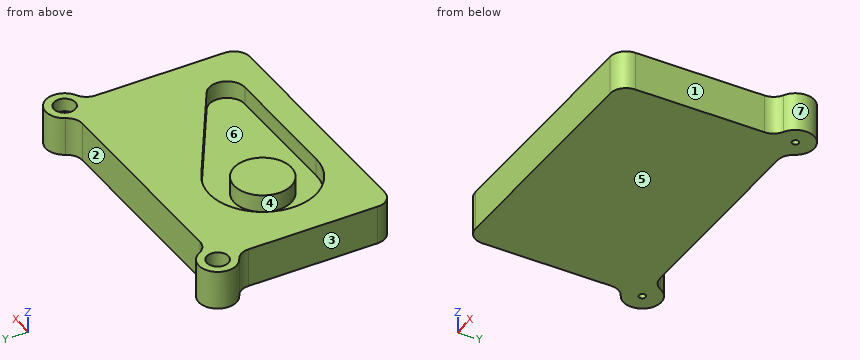
Autodesk Inventor part; units mm, degrees
ref_plane "YZ Plane" through (0, 0, 0) normal (1, 0, 0) x (0, 1, 0)
ref_plane "XZ Plane" through (0, 0, 0) normal (0, 1, 0) x (-1, 0, 0)
ref_plane "XY Plane" through (0, 0, 0) normal (0, 0, 1) x (1, 0, 0)
sketch "Sketch1" plane through (0, 0, 0) normal (0, 0, 1) x (1, 0, 0)
  line L0 (-85.9222, 66) -> (85.9222, 66)
  line L1 (100, 51.9222) -> (100, -66)
  line L2 (100, -66) -> (-100, -66)
  line L3 (-100, -66) -> (-100, 51.9222)
  line L4 (-100, 66) -> (100, -66) construction
  line L5 (100, 66) -> (-100, -66) construction
  arc A0 (-85.9222, 66) -> (-100, 51.9222) centre (-100, 66) ccw
  arc A1 (100, 51.9222) -> (85.9222, 66) centre (100, 66) ccw
  line L6 (0, 116.2908) -> (0, -96.3818)
  line L7 (-167.8726, 0) -> (167.8726, 0)
  point P0 (0, 0)
  dimension "d0" = 200
  dimension "d1" = 132
  dimension "d3" = 28.1556
  dimension "d35" = 200
extrude "Extrusion1" add sketch "Sketch1" along normal blind 29.2
fillet "Fillet1" radius 12 6 edges at (-85.9222, 66, 14.6) (85.9222, 66, 14.6) (-100, 51.9222, 14.6) (-100, -66, 14.6) (100, -66, 14.6) (100, 51.9222, 14.6)
sketch "Sketch2" plane through (0, 0, 29.2) normal (0, 0, 1) x (1, 0, 0)
  arc A0 (-87.5012, 72.4781) -> (-106.4781, 53.5012) centre (-100, 66) ccw
  circle A1 centre (-33.4, -6) radius 21.33
  arc A2 (-12.2198, 27.9323) -> (-33.4, -46) centre (-33.4, -6) ccw
  arc A3 (59.8, -46) -> (66.8424, -21.4175) centre (59.8, -32.7) ccw
  line L0 (-33.4, -46) -> (59.8, -46)
  line L1 (66.8424, -21.4175) -> (-12.2198, 27.9323)
  point P0 (-88, -66)
  point P1 (0, 0)
  dimension "d7" = 42.66
  dimension "d8" = 60
  dimension "d9" = 66.6
  dimension "d10" = 80
  dimension "d12" = 93.2
  dimension "d13" = 26.6
extrude "Extrusion2" cut sketch "Sketch2" against normal blind 13.2
hole "Hole1" at (-100, 66, 29.2) direction (0, 0, -1) diameter 5 end through all counterbore diameter 16 counterbore depth 13.2
hole "Hole2" at (100, 66, 29.2) direction (0, 0, -1) diameter 5 end through all counterbore diameter 16 counterbore depth 10
equation "\"d1\" = 0.66 * d0"
equation "\"d3\" = 0.2133 * d1"
equation "\"d35\" = d0"
equation "\"d4\" = 0.146 * d0"
equation "\"d6\" = 0.06 * d0"
equation "\"d7\" = 0.2133 * d0"
equation "\"d9\" = 0.333 * d0"
equation "\"d10\" = 0.4 * d0"
equation "\"d12\" = 0.466 * d0"
equation "\"d13\" = 0.133 * d0"
equation "\"d15\" = 0.066 * d0"
equation "\"d21\" = 0.08 * d0"
equation "\"d22\" = 0.066 * d0"
equation "\"d30\" = 0.08 * d0"
equation "\"d31\" = 0.05 * d0"
properties part number "Tutorial1"
Verification items for the finished model (mm, model axes). Face numbers are marked on the shaded views. A direction names the side the tool comes from. Coordinates: 2 decimals unless noted, no trailing zeros. Loops run counter-clockwise (first coordinate to the right, second up) from the corner with the lowest first, then second, coordinate; pieces in that order, holes last. Notation, with made-up numbers: (56.25, 31.25) -> (103.25, 31.25) arc R4 cw to (103.25, 37.25) -> close; hole circle Ø6 at (-4, -1). An arc over 180 degrees is marked (long way). Answer as CSV lines item,"result".
1) Depth check by flat-ended pin: pin 1 (9 mm diameter, centred on x = -0.5, z = 10.5, fed in from +Y); pin 2 (21 mm diameter, centred on x = -100, y = 66, fed in from -Z); pin 3 (1.5 mm diameter, centred on x = -55.5, y = -12, fed in from +Z); pin 4 (6 mm diameter, centred on y = 37.5, z = 23, fed in from -X). Enter the tip coordinate at first touch or a pass-through.
Found:
pin 1,"stops at y = 66"
pin 2,"stops at z = 0"
pin 3,"stops at z = 16"
pin 4,"stops at x = -100"
2) Release check for a two-part mould opening along Y. For the marked faces 5, 6 and 7 record: +Y half, -Y half, draft (parallel to the pull), parting line (faces both ways), or undercut.
Found:
face 5,"draft"
face 6,"undercut"
face 7,"parting line"
3) Cross-section at D-D, the plane x = -69. Record the cut outline in (y, z), then the cut area to 3 significant figures.
Found:
outline,"(-66, 0) -> (66, 0) -> (66, 29.2) -> (12.24, 29.2) -> (12.24, 16) -> (-24.24, 16) -> (-24.24, 29.2) -> (-66, 29.2) -> close"
area,"3,370 mm2"
4) Tool access check on the marked faces 1, 2, 3 and 4. Record the directions out of +Z, -Z, +X, -X, +Y, -Y that give a thin tool (end or side, any length) a straight path to the whole face; none if there is none.
Found:
face 1,"+Z, -Z, +X, -Y"
face 2,"+Z, -Z, +Y"
face 3,"+Z, -Z, -X, -Y"
face 4,"+Z"
5) Cross-section at B-B, the plane x = 3. Record the cut outline in (y, z), then the cut area to 3 significant figures.
Found:
outline,"(-66, 0) -> (66, 0) -> (66, 29.2) -> (18.43, 29.2) -> (18.43, 16) -> (-46, 16) -> (-46, 29.2) -> (-66, 29.2) -> close"
area,"3,000 mm2"
6) Thickness scan on L1, parallel to Y at x = -17, z = 20.5; L2, parallel to X at y = 5.5, z = 20.5; L3, parallel to Z at x = -45, y = 22.5. Record the ranges inside material, lowest first. Write a range as from..to.
Found:
L1,"y = -66..-46, -19.64..7.64, 30.48..66"
L2,"x = -100..-71.71, -51.36..-15.44, 23.72..100"
L3,"z = 0..16"
7) Cross-section at A-A, the plane z = 21.5. Record the cut outline in (x, y).
Found:
outline,"(-106.48, 53.5) arc R12 cw to (-100, 42.85) -> (-100, -54) arc R12 ccw to (-88, -66) -> (88, -66) arc R12 ccw to (100, -54) -> (100, 42.85) arc R12 cw to (106.48, 53.5) arc R14.08 ccw (long way) to (87.5, 72.48) arc R12 cw to (76.85, 66) -> (-76.85, 66) arc R12 cw to (-87.5, 72.48) arc R14.08 ccw (long way) to start; circle Ø42.66 at (-33.4, -6); hole circle Ø16 at (-100, 66); hole (-33.4, -46) -> (59.8, -46) arc R13.3 ccw to (66.84, -21.42) -> (-12.22, 27.93) arc R40 ccw (long way) to start; hole circle Ø16 at (100, 66)"
8) Cross-section at C-C, the plane y = -6. Record the cut outline in (x, z), then the cut area to 3 significant figures.
Found:
outline,"(-100, 0) -> (100, 0) -> (100, 29.2) -> (42.14, 29.2) -> (42.14, 16) -> (-12.07, 16) -> (-12.07, 29.2) -> (-54.73, 29.2) -> (-54.73, 16) -> (-73.4, 16) -> (-73.4, 29.2) -> (-100, 29.2) -> close"
area,"4,880 mm2"
